Drawing for the job (mm, zero at the part's lowest x, y, z). A direction names the side the tool comes from. Give positions to 0.01 mm unless a question says otherwise; leave off trailing zeros. Order: outer loops, then holes, each group sorted by start corner. A loop starts at its lowest first (then second) coordinate and runs counter-clockwise, first axis right, second up. Notation, with made-up numbers: (18.5, 18) - (61.5, 18) arc R30 cw to (61.5, 49) - close; hole circle Ø8 at (54.25, -21.75). An arc over 180 degrees is marked (long way). One line per item, written item: value.
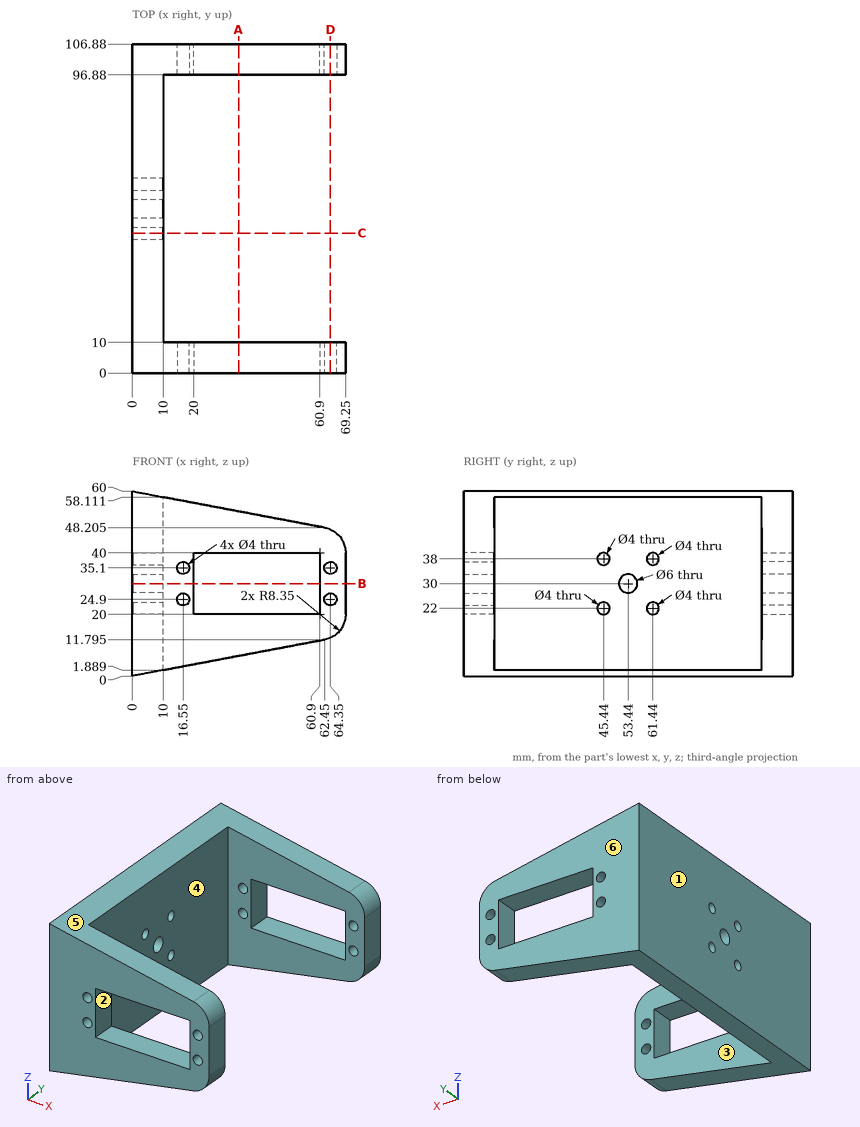
(1) Slice it at C-C, the plane y = 45.44. Give the cut face in (x, z).
Completed:
outline: (0, 0) - (10, 1.89) - (10, 20) - (0, 20) - close; (0, 24) - (10, 24) - (10, 36) - (0, 36) - close; (0, 40) - (10, 40) - (10, 58.11) - (0, 60) - close
(2) Slice it at B-B, the plane z = 30. Give the cut face in (x, y), and give its area (3 significant figures).
Completed:
outline: (0, 0) - (20, 0) - (20, 10) - (10, 10) - (10, 50.44) - (0, 50.44) - close; (0, 56.44) - (10, 56.44) - (10, 96.88) - (20, 96.88) - (20, 106.88) - (0, 106.88) - close; (60.9, 0) - (69.25, 0) - (69.25, 10) - (60.9, 10) - close; (60.9, 96.88) - (69.25, 96.88) - (69.25, 106.88) - (60.9, 106.88) - close
area: 1,380 mm²
(3) Slice it at D-D, the plane x = 64.35. Give the cut face in (y, z).
Completed:
outline: (0, 12.4) - (10, 12.4) - (10, 22.9) - (0, 22.9) - close; (0, 26.9) - (10, 26.9) - (10, 33.1) - (0, 33.1) - close; (0, 37.1) - (10, 37.1) - (10, 47.6) - (0, 47.6) - close; (96.88, 12.4) - (106.88, 12.4) - (106.88, 22.9) - (96.88, 22.9) - close; (96.88, 26.9) - (106.88, 26.9) - (106.88, 33.1) - (96.88, 33.1) - close; (96.88, 37.1) - (106.88, 37.1) - (106.88, 47.6) - (96.88, 47.6) - close
(4) Drill centre lines: line 1 (Y direction, x = 62, z = 42.5); line 2 (Z direction, x = 64.35, y = 102.25) (1 decimal); line 3 (Z direction, x = 16, y = 100). Where is each one in solid material? Low to high.
Completed:
line 1: 0 to 10, 96.88 to 106.88
line 2: 12.4 to 22.9, 26.9 to 33.1, 37.1 to 47.6
line 3: 3.02 to 22.98, 26.82 to 33.18, 37.02 to 56.98
(5) Slice it at A-A, the plane x = 34.5. Give the cut face in (y, z).
Completed:
outline: (0, 6.52) - (10, 6.52) - (10, 20) - (0, 20) - close; (0, 40) - (10, 40) - (10, 53.48) - (0, 53.48) - close; (96.88, 6.52) - (106.88, 6.52) - (106.88, 20) - (96.88, 20) - close; (96.88, 40) - (106.88, 40) - (106.88, 53.48) - (96.88, 53.48) - close
(6) Pin check, flat tips, straight feed: P1, Ø3, axis at x = 21, z = 10, coming from the -Y side; P2, Ø5, axis at x = 46, y = 4.5, coming from the -Z side; P3, Ø8, axis at x = 7.5, y = 96, coming from the -Z side; P4, Ø3, axis at x = 48, y = 100, coming from the +Z side. Stop position of each tip, or through.
Completed:
P1: y = 0
P2: z = 8.22
P3: z = 0.66
P4: z = 51.22
(7) 3-axis set-ups, long thin cutter, end or side, ignore diameter. For the marked faces 1, 2 and 3: which of +Z, -Z, +X, -X, +Y, -Y reach the whole face in a straight line?
Completed:
face 1: +Z, -Z, -X, +Y, -Y
face 2: +Y, -Y
face 3: +Z, -Z, +X
(8) Pull direction Y, two halves, no side cores. Call the marked faces 4, 5 and 6: +Y half, -Y half, draft (parallel to the pull), parting line (faces both ways), or undercut.
Completed:
face 4: undercut
face 5: draft
face 6: +Y half
